Input: part model. Units: mm. Frame: model coordinates. Face numbers are marked on the shaded views. A direction names the side the tool comes from. Round coordinates to 2 decimals unless told otherwise and drop trailing zeros. Order: outer loops, then holes, each group sorted by start corner. A loop starts at its lowest first (then second) coordinate and runs counter-clockwise, first axis right, second up. Notation, with made-up numbers: (-23, 79) - (2, 79) arc R29 cw to (2, 107) - close; hole circle Ø11 at (70, -20). An arc over 180 degrees is marked (long way). One line per item, written item: value. Start each with the question number.
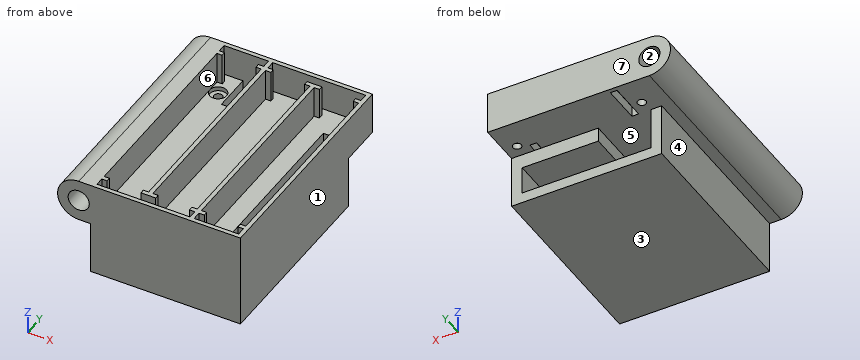
from build123d import *

# Parameters (mm, degrees)
SKETCH1_W           = 30.5
SKETCH1_H           = 10
BOSS_EXTRUDE1_DEPTH = 2.5
SKETCH2_W           = 35.5
SKETCH2_H           = 15
BOSS_EXTRUDE3_DEPTH = 45
SKETCH3_W           = 7.5
SKETCH3_H           = 3.4
CUT_EXTRUDE1_DEPTH  = 29
SKETCH4_W           = 35.5
SKETCH4_H           = 2.5
BOSS_EXTRUDE4_DEPTH = 10
SKETCH5_W           = 35.5
SKETCH5_H           = 55
SKETCH5_W_2         = 33.5
SKETCH5_H_2         = 53
BOSS_EXTRUDE5_DEPTH = 7.5
SKETCH6_W           = 10.5
SKETCH6_H           = 47
BOSS_EXTRUDE6_DEPTH = 7.5
SKETCH7_W           = 8
SKETCH7_H           = 1
SKETCH7_W_2         = 1
SKETCH7_H_2         = 2
CUT_EXTRUDE2_DEPTH  = 7.5
SKETCH8_W           = 1.6
SKETCH8_H           = 46
SKETCH8_H_2         = 9
CUT_EXTRUDE3_DEPTH  = 2.5
CUT_EXTRUDE4_REACH  = 17
SKETCH9_R           = 1
SKETCH10_R          = 2
CUT_EXTRUDE5_DEPTH  = 1
SKETCH11_R          = 2.5
BOSS_EXTRUDE8_DEPTH = 55


with BuildPart() as part:
    # Sketch1 → Boss-Extrude1 (new body)
    with BuildSketch(Plane(origin=(0, 0, 0), x_dir=(1, 0, 0), z_dir=(0, 1, 0))):
        Rectangle(SKETCH1_W, SKETCH1_H)
    extrude(amount=BOSS_EXTRUDE1_DEPTH)

    # Sketch2 → Boss-Extrude3 (add)
    with BuildSketch(Plane(origin=(0, 0, 0), x_dir=(1, 0, 0), z_dir=(0, 1, 0))):
        Rectangle(SKETCH2_W, SKETCH2_H)
        Polygon((-15.25, 5), (-15.25, -5), (-10.25, -5), (-10.25, -1.6), (15.25, -1.6), (15.25, 5), align=None, mode=Mode.SUBTRACT)
    extrude(amount=BOSS_EXTRUDE3_DEPTH)

    # Sketch3 → Cut-Extrude1 (cut)
    with BuildSketch(Plane(origin=(0, 45, 0), x_dir=(1, 0, 0), z_dir=(0, 1, 0))):
        with Locations((-6.5, -3.3)):
            Rectangle(SKETCH3_W, SKETCH3_H)
    extrude(amount=-CUT_EXTRUDE1_DEPTH, mode=Mode.SUBTRACT)

    # Sketch4 → Boss-Extrude4 (add)
    with BuildSketch(Plane(origin=(0, 45, 0), x_dir=(1, 0, 0), z_dir=(0, 1, 0))):
        with Locations((0, -6.25)):
            Rectangle(SKETCH4_W, SKETCH4_H)
    extrude(amount=BOSS_EXTRUDE4_DEPTH)

    # Sketch5 → Boss-Extrude5 (add)
    with BuildSketch(Plane.XY.offset(7.5)):
        with Locations((0, 27.5)):
            Rectangle(SKETCH5_W, SKETCH5_H)
        with Locations((0, 27.5)):
            Rectangle(SKETCH5_W_2, SKETCH5_H_2, mode=Mode.SUBTRACT)
    extrude(amount=BOSS_EXTRUDE5_DEPTH)

    # Sketch6 → Boss-Extrude6 (add)
    with BuildSketch(Plane.XY.offset(7.5)):
        Polygon((-6.25, 54), (-6.25, 52), (-16.75, 52), (-16.75, 51), (-6.25, 51), (-6.25, 4), (-16.75, 4), (-16.75, 3), (-6.25, 3), (-6.25, 1), (-5.25, 1), (-5.25, 3), (5.25, 3), (5.25, 1), (6.25, 1), (6.25, 3), (16.75, 3), (16.75, 4), (6.25, 4), (6.25, 51), (16.75, 51), (16.75, 52), (6.25, 52), (6.25, 54), (5.25, 54), (5.25, 52), (-5.25, 52), (-5.25, 54), align=None)
        with Locations((0, 27.5)):
            Rectangle(SKETCH6_W, SKETCH6_H, mode=Mode.SUBTRACT)
    extrude(amount=BOSS_EXTRUDE6_DEPTH)

    # Sketch7 → Cut-Extrude2 (cut)
    with BuildSketch(Plane.XY.offset(15)):
        with Locations((0, 51.5)):
            Rectangle(SKETCH7_W, SKETCH7_H)
        with Locations((-11.5, 51.5)):
            Rectangle(SKETCH7_W, SKETCH7_H)
        with Locations((11.5, 51.5)):
            Rectangle(SKETCH7_W, SKETCH7_H)
        with Locations((11.5, 3.5)):
            Rectangle(SKETCH7_W, SKETCH7_H)
        with Locations((5.75, 53)):
            Rectangle(SKETCH7_W_2, SKETCH7_H_2)
        with Locations((0, 3.5)):
            Rectangle(SKETCH7_W, SKETCH7_H)
        with Locations((-11.5, 3.5)):
            Rectangle(SKETCH7_W, SKETCH7_H)
        with Locations((-5.75, 2)):
            Rectangle(SKETCH7_W_2, SKETCH7_H_2)
    extrude(amount=-CUT_EXTRUDE2_DEPTH, mode=Mode.SUBTRACT)

    # Sketch8 → Cut-Extrude3 (cut)
    with BuildSketch(Plane.XY.offset(7.5)):
        with Locations((11.5, 24)):
            Rectangle(SKETCH8_W, SKETCH8_H)
        with Locations((-11.5, 49.5)):
            Rectangle(SKETCH8_W, SKETCH8_H_2)
    extrude(amount=-CUT_EXTRUDE3_DEPTH, mode=Mode.SUBTRACT)

    # Sketch9 → Cut-Extrude4 (cut, up to next)
    with BuildSketch(Plane.XY.offset(7.5), mode=Mode.PRIVATE) as cut_extrude4_sk1:
        with Locations((-14.75, 48)):
            Circle(SKETCH9_R)
    cut_extrude4_tool1 = extrude(cut_extrude4_sk1.sketch, amount=-CUT_EXTRUDE4_REACH, mode=Mode.PRIVATE) & part.part
    add(cut_extrude4_tool1.solids().sort_by_distance((-14.75, 48, 7.5))[0], mode=Mode.SUBTRACT)
    # Sketch9 → Cut-Extrude4 (cut, up to next)
    with BuildSketch(Plane.XY.offset(7.5), mode=Mode.PRIVATE) as cut_extrude4_sk2:
        with Locations((14.75, 48)):
            Circle(SKETCH9_R)
    cut_extrude4_tool2 = extrude(cut_extrude4_sk2.sketch, amount=-CUT_EXTRUDE4_REACH, mode=Mode.PRIVATE) & part.part
    add(cut_extrude4_tool2.solids().sort_by_distance((14.75, 48, 7.5))[0], mode=Mode.SUBTRACT)

    # Sketch10 → Cut-Extrude5 (cut)
    with BuildSketch(Plane.XY.offset(7.5)):
        with Locations((-14.75, 48)):
            Circle(SKETCH10_R)
        with Locations((14.75, 48)):
            Circle(SKETCH10_R)
    extrude(amount=-CUT_EXTRUDE5_DEPTH, mode=Mode.SUBTRACT)

    # Sketch11 → Boss-Extrude8 (add)
    with BuildSketch(Plane(origin=(0, 55, 0), x_dir=(1, 0, 0), z_dir=(0, 1, 0))):
        with BuildLine():
            Line((-17.75, -5), (-20.5, -5))
            ThreePointArc((-20.5, -5), (-25.5, -10), (-20.5, -15))
            Line((-20.5, -15), (-17.75, -15))
            Line((-17.75, -15), (-17.75, -5))
        make_face()
        with Locations((-20.5, -10)):
            Circle(SKETCH11_R, mode=Mode.SUBTRACT)
    extrude(amount=-BOSS_EXTRUDE8_DEPTH)


solid = part.part
Item 1: Section query D-D on z = -3.75. Return loops of the section in (x, y), and give its area (3 significant figures).
Item 2: Pull-direction query (Z, two-part tool) for the marked faces 1, 2 and 3; classes: released by +Z, released by -Z, zero draft, split by the parting line, or undercut.
Item 3: Section query A-A on z = 10. Give the number of separate pieces and of enclosed holes in the cut face, and give its area (3 significant figures).
Item 4: Reachability of the marked faces 4, 5, 6 and 7 from +Z, -Z, +X, -X, +Y, -Y: full face, straight path, thin tool, end or side. Return the list, or none.
Item 5: Section query C-C on x = -19.5. Return loops of the section in (y, z), and give its area (3 significant figures).
Item 6: Line query: L1, parallel to X at y = 37, z = 10; L2, parallel to Y at x = -10, z = 14; L3, parallel to Z at x = -3, y = 7.5. Output: solid intervals per line, ascending.
Item 7: First-contact query: pin 1 Ø1.5 at (x, y) = (1, 45) entering from +Z; pin 2 Ø1 at (x, z) = (-5, 2.5) entering from +Y; pin 3 Ø1.5 at (x, z) = (-4.5, -1) entering from +Y. Flat tips, straight axial feed; report the tip coordinate or a pass-through.
Geometry results:
1. outline: (-17.75, 0) - (17.75, 0) - (17.75, 45) - (15.25, 45) - (15.25, 2.5) - (-15.25, 2.5) - (-15.25, 45) - (-17.75, 45) - close
1. area: 301 mm^2
2. face 1: zero draft
2. face 2: undercut
2. face 3: released by -Z
3. separate pieces: 2
3. enclosed holes: 1
3. area: 445 mm^2
4. face 4: -Z, -X, +Y, -Y
4. face 5: +Y
4. face 6: +Z
4. face 7: +Z, -Z, +X, -X, +Y
5. outline: (0, 5) - (55, 5) - (55, 7.71) - (0, 7.71) - close; (0, 12.29) - (55, 12.29) - (55, 15) - (0, 15) - close
5. area: 298 mm^2
6. L1: x = -25.5 to -23, -18 to -16.75, -6.25 to -5.25, 5.25 to 6.25, 16.75 to 17.75
6. L2: y = 0 to 1, 54 to 55
6. L3: z = -7.5 to -5, 1.6 to 7.5
7. pin 1: stops at z = 7.5
7. pin 2: stops at y = 16
7. pin 3: stops at y = 2.5
